```python
from build123d import *

# Parameters (mm, degrees)
BOSS_EXTRU_1_DEPTH             = 3
ENL_V_START                    = -1
ENL_V_MAT_EXTRU_4_DEPTH        = 8.95
BOSS_EXTRU_2_REACH             = 8.95
ESQUISSE4_W                    = 0.7
ESQUISSE4_H                    = 0.5
BOSS_EXTRU_2_DIRECTION_2_DEPTH = 4


with BuildPart() as part:
    # Esquisse1 → Boss.-Extru.1 (new body, symmetric)
    with BuildSketch(Plane(origin=(0, 0, 0), x_dir=(0, 0, -1), z_dir=(1, 0, 0))):
        Polygon((0, 6.95), (1.8, 6.72898779), (1.8, 0.22101221), (0, 0), (-2.1, 0.22101221), (-2.3, 0.242060991), (-2.3, 1.65), (-2.1, 1.85), (-2.1, 6.72898779), align=None)
    extrude(amount=BOSS_EXTRU_1_DEPTH, both=True)

    # Esquisse2 → Enlèv. mat.-Extru.4 (cut)
    with BuildSketch(Plane(origin=(0, 0, 0), x_dir=(1, 0, 0), z_dir=(0, 1, 0)).offset(ENL_V_START)):
        Polygon((0.22814949, -26.29116777), (-2.71759551, -2.3), (-3, 0), (-2.77898779, 1.8), (0.16675721, 25.79116777), (-48.17588371, 25.734183671), (-48.11449143, -26.348151869), align=None)
    enl_v_mat_extru_4 = extrude(amount=ENL_V_MAT_EXTRU_4_DEPTH, mode=Mode.SUBTRACT)

    # Esquisse3 → Révolution1 (revolve)
    with BuildSketch(Plane(origin=(0, 4.3, 0), x_dir=(-1, 0, 0), z_dir=(0, 1, 0))):
        with BuildLine():
            Line((0, 2.1), (2.368543856, 2.1))
            ThreePointArc((2.368543856, 2.1), (1.457737974, 3.331009601), (0, 3.8))
            Line((0, 3.8), (0, 2.1))
        make_face()
    revolve(axis=Axis((0, 4.3, 2.1), (0, 0, 1)))

    # Symétrie1: Enlèv. mat.-Extru.4 across plane
    add(enl_v_mat_extru_4.mirror(Plane(origin=(0, 0, 0), x_dir=(0, 0, 1), z_dir=(1, 0, 0))), mode=Mode.SUBTRACT)

    # Esquisse4 → Boss.-Extru.2 (add, up to next)
    with BuildSketch(Plane(origin=(0, 0, 0), x_dir=(1, 0, 0), z_dir=(0, 1, 0)), mode=Mode.PRIVATE) as boss_extru_2_sk1:
        with Locations((0, 0.25)):
            Rectangle(ESQUISSE4_W, ESQUISSE4_H)
    boss_extru_2_tool1 = extrude(boss_extru_2_sk1.sketch, amount=BOSS_EXTRU_2_REACH, mode=Mode.PRIVATE) - part.part
    add(boss_extru_2_tool1.solids().sort_by_distance((0, 0, -0.25))[0])
    # Esquisse4 → Boss.-Extru.2 (add, up to next)
    with BuildSketch(Plane(origin=(0, 0, 0), x_dir=(1, 0, 0), z_dir=(0, 1, 0)), mode=Mode.PRIVATE) as boss_extru_2_sk2:
        with Locations((2.54, 0.25)):
            Rectangle(ESQUISSE4_W, ESQUISSE4_H)
    boss_extru_2_tool2 = extrude(boss_extru_2_sk2.sketch, amount=BOSS_EXTRU_2_REACH, mode=Mode.PRIVATE) - part.part
    add(boss_extru_2_tool2.solids().sort_by_distance((2.54, 0, -0.25))[0])
    # Esquisse4 → Boss.-Extru.2 (add, up to next)
    with BuildSketch(Plane(origin=(0, 0, 0), x_dir=(1, 0, 0), z_dir=(0, 1, 0)), mode=Mode.PRIVATE) as boss_extru_2_sk3:
        with Locations((-2.54, 0.25)):
            Rectangle(ESQUISSE4_W, ESQUISSE4_H)
    boss_extru_2_tool3 = extrude(boss_extru_2_sk3.sketch, amount=BOSS_EXTRU_2_REACH, mode=Mode.PRIVATE) - part.part
    add(boss_extru_2_tool3.solids().sort_by_distance((-2.54, 0, -0.25))[0])

    # Esquisse4 → Boss.-Extru.2 direction 2 (add)
    with BuildSketch(Plane(origin=(0, 0, 0), x_dir=(1, 0, 0), z_dir=(0, 1, 0))):
        with Locations((0, 0.25)):
            Rectangle(ESQUISSE4_W, ESQUISSE4_H)
        with Locations((2.54, 0.25)):
            Rectangle(ESQUISSE4_W, ESQUISSE4_H)
        with Locations((-2.54, 0.25)):
            Rectangle(ESQUISSE4_W, ESQUISSE4_H)
    extrude(amount=-BOSS_EXTRU_2_DIRECTION_2_DEPTH)


solid = part.part
```
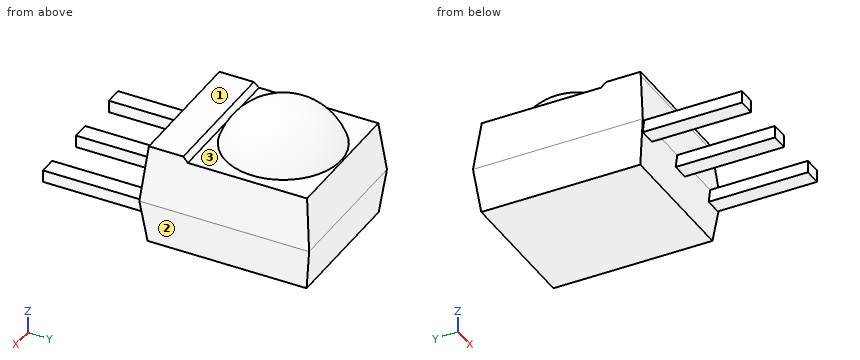
Could you check a few things on this model? Use its own coordinates, in mm. Face numbers are marked on the shaded views. A direction names the side the tool comes from. Round coordinates to 2 decimals unless told otherwise and drop trailing zeros. Loops run counter-clockwise (first coordinate to the right, second up) from the corner with the lowest first, then second, coordinate; pieces in that order, holes last. Notation, with made-up numbers: (38.25, 9.25) -> (43.25, 9.25) arc R13 ccw to (43.25, 17.25) -> close; hole circle Ø11 at (81, -13.75). An arc over 180 degrees is marked (long way). One line per question, with ' | ' between items.
(1) If I drill on probe 1 along Z at (x, y) = (1.25, 2.25); probe 2 along Z at (x, y) = (2.75, -2.75); probe 3 along X at (y, z) = (3, 0.2), over which ranges is the centre line in solid material (lowest first)?
Model answer:
probe 1: z = -1.8 to 2.1 | probe 2: z = -0.5 to 0 | probe 3: x = -2.98 to 2.98
(2) For the marked faces 1, 2 and 3, which set-ups out of +Z, -Z, +X, -X, +Y, -Y let a thin tool reach every point of the face, with its end or its side?
Model answer:
face 1: +Z, +X, -X, -Y | face 2: -Z, +X, +Y, -Y | face 3: +Z
(3) If we section it at B-B on x = 2.5: List the corners of the cut face in (y, z) for me, and give its area (3 significant figures).
Model answer:
outline: (-4, -0.5) -> (0.06, -0.5) -> (0.22, -1.8) -> (6.73, -1.8) -> (6.95, 0) -> (6.73, 2.1) -> (1.85, 2.1) -> (1.65, 2.3) -> (0.24, 2.3) -> (0, 0) -> (-4, 0) -> close | area: 28.6 mm^2
(4) If we section it at C-C on y = 3.75: List the corners of the cut face in (x, z) for me.
Model answer:
outline: (-3, 0) -> (-2.78, -1.8) -> (2.78, -1.8) -> (3, 0) -> (2.74, 2.1) -> (2.3, 2.1) arc R2.44 ccw to (-2.3, 2.1) -> (-2.74, 2.1) -> close
(5) For pin 1 Ø0.8 at (x, y) = (-2.5, -3) entering from +Z; pin 2 Ø1.5 at (y, z) = (2, 1) entering from -X; pin 3 Ø1.5 at (x, y) = (1, 1) entering from +Z, each with a flat end and sliding along its axis, tell me the tip position at first contact or that it passes through.
Model answer:
pin 1: stops at z = 0 | pin 2: stops at x = -2.97 | pin 3: stops at z = 2.3
(6) If we section it at A-A on y = -1: List the corners of the cut face in (x, z) for me.
Model answer:
outline: (-2.89, -0.5) -> (-2.19, -0.5) -> (-2.19, 0) -> (-2.89, 0) -> close; (-0.35, -0.5) -> (0.35, -0.5) -> (0.35, 0) -> (-0.35, 0) -> close; (2.19, -0.5) -> (2.89, -0.5) -> (2.89, 0) -> (2.19, 0) -> close
(7) If we section it at D-D on z = -0.65: List the corners of the cut face in (x, y) for me.
Model answer:
outline: (-2.92, 0.08) -> (2.92, 0.08) -> (2.92, 6.87) -> (-2.92, 6.87) -> close
